Could you check a few things on this model? Use its own coordinates, in mm. Give positions to 0.01 mm unless a question says otherwise; leave off trailing zeros. Order: outer loops, then holes, each group sorted by start corner. A loop starts at its lowest first (then second) coordinate and runs counter-clockwise, first axis right, second up. Notation, with made-up numbers: M 27.25,59 L 34.25,59 A25 ccw 34.25,77 Z; hole C 22.5,16 d6. An arc over 180 degrees is marked long. Use a Markdown table: item, result. Add a question column.
Item 1: I'm going to push a flat-ended pin straight in: pin 1 Ø1.6 at (x, y) = (50, -1) entering from -Z. Where does the tip first touch, or does it pass through?
Item 2: Suppose I cut it at D-D on z = -10. Write out the boundary of the cut face in (x, y) (3 decimals), plus the area to 3 significant figures.
Item 3: Suppose I cut it at C-C on x = -21. Write out the boundary of the cut face in (y, z) (3 decimals), plus the area to 3 significant figures.
Item 4: Suppose I cut it at B-B on z = 14.5. Write out the boundary of the cut face in (x, y) (3 decimals).
Item 5: If I drill on L1, parallel to Z at x = 52.5, y = -0.45; L2, parallel to X at y = -0.65, z = -70.5; L3, parallel to Z at x = 69, y = -2.35, over which ranges is the centre line in solid material (lowest first)? Write a range as from..to.
Item 6: Suppose I cut it at A-A on x = 18.5. Write out the boundary of the cut face in (y, z) (3 decimals), plus the area to 3 significant figures.
from build123d import *

# Parameters (mm, degrees)
SKETCH1_W                    = 127
SKETCH1_H                    = 127
BOSS_EXTRUDE1_DEPTH          = 3.175
M20_CLEARANCE_HOLE1_D        = 22.225
M6_CLEARANCE_HOLE1_D         = 6.7056
HOLE1_D                      = 31.75
M10_CLEARANCE_HOLE1_D        = 11.1252
FILLET1_R                    = 0.79375
M6_CLEARANCE_HOLE2_D         = 6.4
CUT_EXTRUDE1_DEPTH           = 110.992087544
F_3_8_0_375_DIAMETER_HOLE1_D = 9.525


with BuildPart() as part:
    # Sketch1 → Boss-Extrude1 (new body)
    with BuildSketch(Plane(origin=(0, 0, 0), x_dir=(1, 0, 0), z_dir=(0, 1, 0))):
        with Locations((13.673098237, 14.8102267)):
            Rectangle(SKETCH1_W, SKETCH1_H)
    extrude(amount=-BOSS_EXTRUDE1_DEPTH)

    # M20 Clearance Hole1 (through all)
    with Locations(Plane.XZ.offset(3.175)):
        with Locations((13.673098237, 5.5351733)):
            Hole(M20_CLEARANCE_HOLE1_D / 2)

    # M6 Clearance Hole1 (through all)
    with Locations(Plane.XZ.offset(3.175)):
        with Locations((-41.889401763, -70.3727267), (69.235598237, 40.7522733), (69.235598237, -70.3727267), (-41.889401763, 40.7522733)):
            Hole(M6_CLEARANCE_HOLE1_D / 2)

    # Hole1 (through all)
    with Locations(Plane.XZ.offset(3.175)):
        with Locations((13.673098237, -35.1556267)):
            Hole(HOLE1_D / 2)

    # M10 Clearance Hole1 (through all)
    with Locations(Plane.XZ.offset(3.175)):
        with Locations((-24.535146731, -33.8602267), (51.881343204, 16.9397733), (-24.535146731, -8.4602267), (-24.535146731, 16.9397733), (51.881343204, -33.8602267), (51.881343204, -8.4602267)):
            Hole(M10_CLEARANCE_HOLE1_D / 2)

    # Fillet1
    fillet1_edges = [part.edges().sort_by_distance(p)[0] for p in [
        (77.173098237, -1.5875, -78.3102267),
        (77.173098237, -1.5875, 48.6897733),
        (-49.826901763, -1.5875, 48.6897733),
        (-49.826901763, -1.5875, -78.3102267),
    ]]
    fillet(fillet1_edges, radius=FILLET1_R)

    # M6 Clearance Hole2 (through all)
    with Locations(Plane(origin=(0, 0, 0), x_dir=(-1, 0, 0), z_dir=(0, 1, 0))):
        with Locations((-64.473098237, -35.1556267), (37.126901763, -35.1556267)):
            Hole(M6_CLEARANCE_HOLE2_D / 2)

    # Sketch12 → Cut-Extrude1 (cut, through all)
    with BuildSketch(Plane.XZ.offset(3.175)):
        with BuildLine():
            Line((-33.316901763, -78.3102267), (-33.316901763, -61.7462517))
            ThreePointArc((-33.316901763, -61.7462517), (-32.386965793, -59.50118767), (-30.141901763, -58.5712517))
            Line((-30.141901763, -58.5712517), (-7.916901763, -58.5712517))
            ThreePointArc((-7.916901763, -58.5712517), (-5.671837733, -59.50118767), (-4.741901763, -61.7462517))
            Line((-4.741901763, -61.7462517), (-4.741901763, -78.3102267))
            Line((-4.741901763, -78.3102267), (-33.316901763, -78.3102267))
        make_face()
        with BuildLine():
            Line((32.075398237, -78.3102267), (32.075398237, -61.7462517))
            ThreePointArc((32.075398237, -61.7462517), (33.005334207, -59.50118767), (35.250398237, -58.5712517))
            Line((35.250398237, -58.5712517), (57.500798237, -58.5712517))
            ThreePointArc((57.500798237, -58.5712517), (59.745862267, -59.50118767), (60.675798237, -61.7462517))
            Line((60.675798237, -61.7462517), (60.675798237, -78.3102267))
            Line((60.675798237, -78.3102267), (32.075398237, -78.3102267))
        make_face()
    extrude(amount=-CUT_EXTRUDE1_DEPTH, mode=Mode.SUBTRACT)

    # 3/8 (0.375) Diameter Hole1 (through all)
    with Locations(Plane.XZ.offset(3.175)):
        with Locations((60.663098237, 31.717491348), (-33.316901763, 31.717491348)):
            Hole(F_3_8_0_375_DIAMETER_HOLE1_D / 2)


solid = part.part
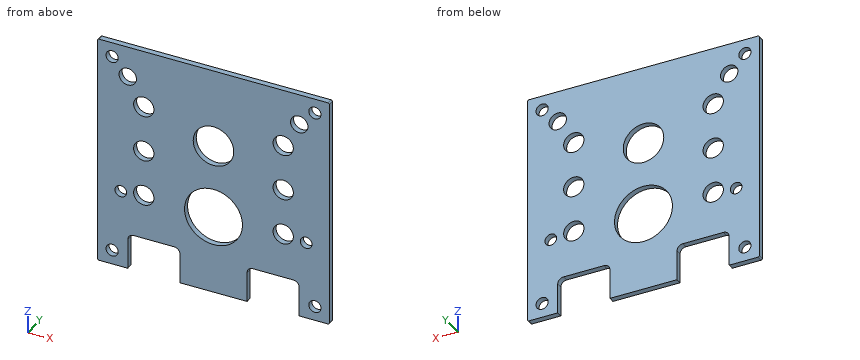
Findings below:
| question | item | result |
|---|---|---|
| 1 | pin 1 | stops at z = -58.57 |
| 2 | outline | M -49.827,-3.175 L -29.88,-3.175 L -29.88,0 L -49.827,0 Z; M -19.19,-3.175 L 46.536,-3.175 L 46.536,0 L -19.19,0 Z; M 57.227,-3.175 L 77.173,-3.175 L 77.173,0 L 57.227,0 Z |
| 2 | area | 335 mm^2 |
| 3 | outline | M -3.175,-58.571 L 0,-58.571 L 0,-38.155 L -3.175,-38.155 Z; M -3.175,-29.565 L 0,-29.565 L 0,-12.755 L -3.175,-12.755 Z; M -3.175,-4.165 L 0,-4.165 L 0,12.645 L -3.175,12.645 Z; M -3.175,21.235 L 0,21.235 L 0,48.69 L -3.175,48.69 Z |
| 3 | area | 259 mm^2 |
| 4 | outline | M -49.827,-3.175 L -29.534,-3.175 L -29.534,0 L -49.827,0 Z; M -19.536,-3.175 L 7.107,-3.175 L 7.107,0 L -19.536,0 Z; M 20.24,-3.175 L 46.882,-3.175 L 46.882,0 L 20.24,0 Z; M 56.88,-3.175 L 77.173,-3.175 L 77.173,0 L 56.88,0 Z |
| 5 | L1 | z = -58.57..-39.39, -28.33..-13.99, -2.93..11.41, 22.47..48.69 |
| 5 | L2 | x = -49.83..-45.24, -38.54..-33.32, -4.74..32.08, 60.68..65.89, 72.59..77.17 |
| 5 | L3 | z = -78.31..-73.72, -67.03..37.41, 44.1..48.69 |
| 6 | outline | M -3.175,-78.31 L 0,-78.31 L 0,-50.279 L -3.175,-50.279 Z; M -3.175,-20.032 L 0,-20.032 L 0,-4.474 L -3.175,-4.474 Z; M -3.175,15.545 L 0,15.545 L 0,48.69 L -3.175,48.69 Z |
| 6 | area | 244 mm^2 |
